```python
from build123d import *

# Parameters (mm, degrees)
SKETCH1_W                    = 158
SKETCH1_H                    = 50
BASE_FLANGE1_DEPTH           = 8
EDGE_FLANGE1_STRIP_W         = 48
EDGE_FLANGE1_STRIP_H         = 8
EDGE_FLANGE1_STRIP_CUT_DEPTH = 158
EDGE_FLANGE1_DEPTH           = 158
CHAMFER1_SIZE                = 40.5
CHAMFER1_SIZE2               = 28.358405297
MIRROR2_START                = 55.822576735
MIRROR2_OUTLINE_W            = 53
MIRROR2_OUTLINE_H            = 13
MIRROR2_DEPTH                = 23.229845673


# Read off the part's stored shape, not the designer's step: Mirror2
# Sheet-metal steps are written as plain solids
with BuildPart() as part:
    # Sketch1 → Base-Flange1 (new body)
    with BuildSketch(Plane(origin=(0, 0, 0), x_dir=(1, 0, 0), z_dir=(0, 1, 0))):
        Rectangle(SKETCH1_W, SKETCH1_H)
    extrude(amount=-BASE_FLANGE1_DEPTH)

    # Edge-Flange1 strip (across the edge) → Edge-Flange1 strip cut (cut)
    with BuildSketch(Plane(origin=(-79, 0, 25), x_dir=(0, 0, -1), z_dir=(1, 0, 0))):
        with Locations((-8, -4)):
            Rectangle(EDGE_FLANGE1_STRIP_W, EDGE_FLANGE1_STRIP_H)
    extrude(amount=EDGE_FLANGE1_STRIP_CUT_DEPTH, mode=Mode.SUBTRACT)

    # Edge-Flange1 section (across the edge) → Edge-Flange1 (add)
    with BuildSketch(Plane(origin=(-79, 0, 25), x_dir=(0, 0, -1), z_dir=(1, 0, 0))):
        with BuildLine():
            Line((0, 8), (0, 32))
            Line((0, 32), (8, 32))
            Line((8, 32), (8, 8))
            ThreePointArc((8, 8), (10.343145751, 2.343145751), (16, 0))
            Line((16, 0), (16, -8))
            ThreePointArc((16, -8), (4.686291501, -3.313708499), (0, 8))
        make_face()
    extrude(amount=EDGE_FLANGE1_DEPTH)

    # Chamfer1
    chamfer1_edges = [part.edges().sort_by_distance(p)[0] for p in [
        (-79, -4, -25),
    ]]
    chamfer1_side = [part.faces().sort_by_distance(p)[0] for p in [
        (-79, -0.640312424, -8),
    ]]
    chamfer(chamfer1_edges, length=CHAMFER1_SIZE, length2=CHAMFER1_SIZE2, reference=chamfer1_side[0])

    # Mirror2 outline → Mirror2 (cut)
    with BuildSketch(Plane(origin=(0, 0, 0), x_dir=(0.5735764363510512, 0, 0.8191520442889882), z_dir=(0.8191520442889882, 0, -0.5735764363510512)).offset(MIRROR2_START)):
        with Locations((33.5, 1.5)):
            Rectangle(MIRROR2_OUTLINE_W, MIRROR2_OUTLINE_H)
    extrude(amount=MIRROR2_DEPTH, mode=Mode.SUBTRACT)


solid = part.part
```
Work out the finished part from the listing and answer in its coordinate system (mm). A direction names the side the tool comes from. Coordinates: 2 decimals unless noted, no trailing zeros. Loops run counter-clockwise (first coordinate to the right, second up) from the corner with the lowest first, then second, coordinate; pieces in that order, holes last. Notation, with made-up numbers: (6.5, 33) - (59.5, 33) arc R21 cw to (59.5, 40) - close; hole circle Ø3 at (39, -11.5). An arc over 180 degrees is marked (long way). Use a Markdown table: item, result.
Item 1: Find section A-A, the plane x = 22. Determine the outline of the cut face in (y, z), and give its area (3 significant figures).
Evaluation:
| item | result |
|---|---|
| outline | (-8, -25) - (0, -25) - (0, 9) arc R8 cw to (8, 17) - (32, 17) - (32, 25) - (8, 25) arc R16 ccw to (-8, 9) - close |
| area | 615 mm2 |
Item 2: Consider probe 1 along Y at (x, z) = (22.5, 6.5); probe 2 along Z at (x, y) = (37, 20); probe 3 along Z at (x, y) = (23, -2.5). Determine where each line is inside the solid, lowest interval first. Write a range as from..to.
Evaluation:
| item | result |
|---|---|
| probe 1 | y = -8..0 |
| probe 2 | z = 17..25 |
| probe 3 | z = -25..21.07 |
Item 3: Find section C-C, the plane z = -1. Determine the outline of the cut face in (x, y).
Evaluation:
| item | result |
|---|---|
| outline | (-67.45, -8) - (67.45, -8) - (67.45, 0) - (-67.45, 0) - close |
Item 4: For faces 1 (the flat face through (-1, 20, 17)), 2 (the flat face through (64.622, -3.671, -5.033)), determine the directions among +Z, -Z, +X, -X, +Y, -Y from which every point of the face is accessible in a straight line to the end or side of a thin tool.
Evaluation:
| item | result |
|---|---|
| face 1 | -Z, +X, -X, +Y |
| face 2 | -Z, +X, +Y, -Y |
Item 5: Given pin 1 Ø4 at (x, z) = (45.5, 3.5) entering from +Y; pin 2 Ø1.5 at (y, z) = (-2, 12.5) entering from +X; pin 3 Ø6 at (x, y) = (10, 6.5) entering from -Z, each flat-ended and moving along its own axis, determine where each tip first touches the part or whether it passes through.
Evaluation:
| item | result |
|---|---|
| pin 1 | stops at y = 0 |
| pin 2 | stops at x = 77.42 |
| pin 3 | stops at z = 15.61 |
Item 6: Find section D-D, the plane y = -4.5. Determine the outline of the cut face in (x, z), and give its area (3 significant figures).
Evaluation:
| item | result |
|---|---|
| outline | (-79, 15.5) - (-50.64, -25) - (50.64, -25) - (79, 15.5) - (79, 18.99) - (-79, 18.99) - close |
| area | 5,800 mm2 |
Item 7: Find section B-B, the plane y = 17. Determine the outline of the cut face in (x, z), and give its area (3 significant figures).
Evaluation:
| item | result |
|---|---|
| outline | (-79, 17) - (79, 17) - (79, 25) - (-79, 25) - close |
| area | 1,260 mm2 |
